```python
from build123d import *

# Parameters (mm, degrees)
SKETCH1_W           = 57.5
SKETCH1_H           = 25
SKETCH1_R           = 4.65
SKETCH1_R_2         = 1.75
BOSS_EXTRUDE1_DEPTH = 3
SKETCH2_W           = 10
SKETCH2_H           = 25
BOSS_EXTRUDE2_DEPTH = 17
SKETCH4_W           = 3
SKETCH4_H           = 25
BOSS_EXTRUDE3_DEPTH = 15
SKETCH8_R           = 69.668681809
SKETCH8_R_2         = 40
CUT_EXTRUDE3_DEPTH  = 40
SKETCH9_R           = 2.625
CUT_EXTRUDE4_DEPTH  = 5
SKETCH11_R          = 34.641133141
SKETCH11_R_2        = 25
CUT_EXTRUDE5_DEPTH  = 17
FILLET1_R           = 5


with BuildPart() as part:
    # Sketch1 → Boss-Extrude1 (new body)
    with BuildSketch(Plane.XY):
        Rectangle(SKETCH1_W, SKETCH1_H)
        Circle(SKETCH1_R, mode=Mode.SUBTRACT)
        with Locations((-10, 0)):
            Circle(SKETCH1_R_2, mode=Mode.SUBTRACT)
    extrude(amount=BOSS_EXTRUDE1_DEPTH)

    # Sketch2 → Boss-Extrude2 (add)
    with BuildSketch(Plane(origin=(0, 0, 0), x_dir=(-1, 0, 0), z_dir=(0, 0, -1))):
        with Locations((-23.75, 0)):
            Rectangle(SKETCH2_W, SKETCH2_H)
    boss_extrude2 = extrude(amount=BOSS_EXTRUDE2_DEPTH)

    # Sketch4 → Boss-Extrude3 (add)
    with BuildSketch(Plane(origin=(28.75, 0, 0), x_dir=(0, 0, -1), z_dir=(1, 0, 0))):
        with Locations((15.5, 0)):
            Rectangle(SKETCH4_W, SKETCH4_H)
    boss_extrude3 = extrude(amount=BOSS_EXTRUDE3_DEPTH)

    # Mirror2: Boss-Extrude2 across plane
    add(boss_extrude2.mirror(Plane(origin=(0, 0, 0), x_dir=(0, 0, 1), z_dir=(1, 0, 0))))

    # Mirror3: Boss-Extrude3 across plane
    add(boss_extrude3.mirror(Plane(origin=(0, 0, 0), x_dir=(0, 0, 1), z_dir=(1, 0, 0))))

    # Sketch8 → Cut-Extrude3 (cut)
    with BuildSketch(Plane(origin=(0, 0, -17), x_dir=(-1, 0, 0), z_dir=(0, 0, -1))):
        Circle(SKETCH8_R)
        Circle(SKETCH8_R_2, mode=Mode.SUBTRACT)
    extrude(amount=-CUT_EXTRUDE3_DEPTH, mode=Mode.SUBTRACT)

    # Sketch9 → Cut-Extrude4 (cut, symmetric)
    with BuildSketch(Plane.XY.offset(-14)):
        with Locations(Location((-33.75, 0, 0), (0, 0, 270))):
            Circle(SKETCH9_R)
        with Locations(Location((33.75, 0, 0), (0, 0, 90))):
            Circle(SKETCH9_R)
    extrude(amount=CUT_EXTRUDE4_DEPTH, both=True, mode=Mode.SUBTRACT)

    # Sketch11 → Cut-Extrude5 (cut)
    with BuildSketch(Plane.XY.offset(3)):
        Circle(SKETCH11_R)
        Circle(SKETCH11_R_2, mode=Mode.SUBTRACT)
    extrude(amount=-CUT_EXTRUDE5_DEPTH, mode=Mode.SUBTRACT)

    # Fillet1
    fillet1_edges = [part.edges().sort_by_distance(p)[0] for p in [
        (-25, 0, -14),
        (25, 0, -14),
        (18.75, 0, 0),
        (-18.75, 0, 0),
    ]]
    fillet(fillet1_edges, radius=FILLET1_R)


solid = part.part
```
The listing builds one solid part. Answer for the finished solid, in the listing's coordinates (mm). A direction names the side the tool comes from. Coordinates: 2 decimals unless noted, no trailing zeros. Write each loop counter-clockwise with the first axis right and the second up, starting at its lowest first coordinate (ties: lowest second). Pieces come first, ordered by that corner, then holes. Notation, with made-up numbers: (27, 62.25) - (48, 62.25) arc R14 ccw to (48, 77.25) - close; hole circle Ø4 at (55.5, 46). An arc over 180 degrees is marked (long way). Return JSON: item names as keys, results as strings. Group by question number.
Q1. The part is cut by section A-A on y = 0. State how many separate pieces and enclosed holes the cut face has, and give its area (3 significant figures).
Q2. The part is cut by section C-C on x = 0. Write down the section's boundary in (y, z), and give its area (3 significant figures).
Q3. The part is cut by section D-D on x = -15.5. Write down the section's boundary in (y, z), and give its area (3 significant figures).
Q4. Find the intervals of material crossed by line 1 along X through (y, z) = (0, -16.15) (3 decimals); line 2 along Y through (x, z) = (-10, 1.7); line 3 along X through (y, z) = (0.75, -8.75), in increasing order. Write a range as [from, to].
Q5. Which of the six approach directions +Z, -Z, +X, -X, +Y, -Y give full straight-line access (tool end or side, diameter ignored) to faces 4 (the cylindrical face through (25, 0, -3)), 5 (the flat face through (-18.75, 0, -11)), 6 (the cylindrical face through (36.313, -0.569, -15.479))?
Q6. For a pull along Y with two mould halves and no side action, classify faces 1 (the flat face through (5, 0, 3)), 2 (the cylindrical face through (-8.331, 0.526, 1.479)), 3 (the cylindrical face through (-25, 0, -3)) as +Y half, -Y half, draft (parallel to the pull), parting line (faces both ways), or undercut.
Q7. The part is cut by section B-B on z = -2. Write down the section's boundary in (x, y), and give its area (3 significant figures).
Q8. Flat-ended cylindrical pins translate along their axes: pin 1 Ø8 at (x, y) = (13.5, -5) entering from -Z; pin 2 Ø9.5 at (y, z) = (-1.5, -8.5) entering from -X; pin 3 Ø2 at (y, z) = (3.5, -7.5) entering from +X; pin 4 Ø4.5 at (x, y) = (-33.75, 0) entering from -Z. Find the tip coordinate at first contact, or state that the pin passes through.
Evaluation:
{
 "1": {"separate pieces": "5", "enclosed holes": "0", "area": "404 mm2"},
 "2": {"outline": "(-12.5, 0) - (-4.65, 0) - (-4.65, 3) - (-12.5, 3) - close; (4.65, 0) - (12.5, 0) - (12.5, 3) - (4.65, 3) - close", "area": "47.1 mm2"},
 "3": {"outline": "(-12.5, -0.32) - (12.5, -0.32) - (12.5, 3) - (-12.5, 3) - close", "area": "82.9 mm2"},
 "4": {"line 1": "x = [-40, -36.375], [-31.125, -18.75], [18.75, 31.125], [36.375, 40]", "line 2": "y = [-12.5, -1.75], [1.75, 12.5]", "line 3": "x = [-24.99, -18.75], [18.75, 24.99]"},
 "5": {"face 4": "+Z, +X", "face 5": "-Z, +Y, -Y", "face 6": "+Z, -Z"},
 "6": {"face 1": "draft", "face 2": "undercut", "face 3": "parting line"},
 "7": {"outline": "(-21.65, -12.5) - (-17.75, -12.5) - (-17.75, 12.5) - (-21.65, 12.5) arc R25 ccw to start; (17.75, -12.5) - (21.65, -12.5) arc R25 ccw to (21.65, 12.5) - (17.75, 12.5) - close", "area": "308 mm2"},
 "8": {"pin 1": "stops at z = -1.69", "pin 2": "stops at x = -27.33", "pin 3": "stops at x = 24.87", "pin 4": "passes through"}
}
